```python
from build123d import *

# Parameters (mm, degrees)
SKETCH1_R           = 16
BOSS_EXTRUDE1_DEPTH = 7
CUT_EXTRUDE1_START  = -5
SKETCH3_R           = 16
SKETCH3_R_2         = 15
CUT_EXTRUDE1_DEPTH  = 5


with BuildPart() as part:
    # Sketch1 → Boss-Extrude1 (new body)
    with BuildSketch(Plane(origin=(0, 0, 0), x_dir=(0, 0, -1), z_dir=(1, 0, 0))):
        Circle(SKETCH1_R)
        with BuildLine():
            Line((-1.923932435, 0.546336878), (1.435107833, 1.393005925))
            ThreePointArc((1.435107833, 1.393005925), (0.488824602, -1.939342803), (-1.923932435, 0.546336878))
        make_face(mode=Mode.SUBTRACT)
    extrude(amount=BOSS_EXTRUDE1_DEPTH)

    # Sketch3 → Cut-Extrude1 (cut)
    with BuildSketch(Plane(origin=(6, 0, 0), x_dir=(0, 0, -1), z_dir=(1, 0, 0)).offset(CUT_EXTRUDE1_START)):
        Circle(SKETCH3_R)
        Circle(SKETCH3_R_2, mode=Mode.SUBTRACT)
    extrude(amount=CUT_EXTRUDE1_DEPTH, mode=Mode.SUBTRACT)


solid = part.part
```
The model under review builds one solid part; all positions refer to its coordinate system, in mm. A direction names the side the tool comes from. Round coordinates to 2 decimals unless told otherwise and drop trailing zeros. Order: outer loops, then holes, each group sorted by start corner. A loop starts at its lowest first (then second) coordinate and runs counter-clockwise, first axis right, second up. Notation, with made-up numbers: (-8.5, 89.5) -> (7.5, 89.5) arc R21 ccw to (7.5, 98.5) -> close; hole circle Ø10 at (28, -33). An arc over 180 degrees is marked (long way). Use a Markdown table: item, result.
Q1. Mouldability with a two-part tool opening along Y and no side actions: class faces 1 (the cylindrical face through (3.451, -1.924, -0.545)), 2 (the cylindrical face through (0.49, -15.62, 3.47)), 3 (the flat face through (7, 0, -3)) as +Y half, -Y half, draft (parallel to the pull), parting line (faces both ways), or undercut.
Values:
| item | result |
|---|---|
| face 1 | undercut |
| face 2 | parting line |
| face 3 | draft |
Q2. We need section C-C on z = 6.5. Write out the cut boundary in (x, y).
Values:
| item | result |
|---|---|
| outline | (0, -14.62) -> (1, -14.62) -> (1, -13.52) -> (6, -13.52) -> (6, -14.62) -> (7, -14.62) -> (7, 14.62) -> (6, 14.62) -> (6, 13.52) -> (1, 13.52) -> (1, 14.62) -> (0, 14.62) -> close |
Q3. We need section A-A on y = 0. Write out the cut boundary in (x, z), then the cut area to 3 significant figures.
Values:
| item | result |
|---|---|
| outline | (0, -16) -> (1, -16) -> (1, -15) -> (6, -15) -> (6, -16) -> (7, -16) -> (7, -2) -> (0, -2) -> close; (0, 2) -> (7, 2) -> (7, 16) -> (6, 16) -> (6, 15) -> (1, 15) -> (1, 16) -> (0, 16) -> close |
| area | 186 mm^2 |
Q4. We need section B-B on z = -1. Write out the cut boundary in (x, y), then the cut area to 3 significant figures.
Values:
| item | result |
|---|---|
| outline | (0, -15.97) -> (1, -15.97) -> (1, -14.97) -> (6, -14.97) -> (6, -15.97) -> (7, -15.97) -> (7, -1.73) -> (0, -1.73) -> close; (0, 1.28) -> (7, 1.28) -> (7, 15.97) -> (6, 15.97) -> (6, 14.97) -> (1, 14.97) -> (1, 15.97) -> (0, 15.97) -> close |
| area | 192 mm^2 |
Q5. For line 1 (X direction, y = -6, z = 14); line 2 (Y direction, x = 4.75, z = 0); line 3 (Z direction, x = 4, y = 9), list the stretches that pass through material, from the lowest coordinate up.
Values:
| item | result |
|---|---|
| line 1 | x = 0 to 1, 6 to 7 |
| line 2 | y = -15 to -2, 1.03 to 15 |
| line 3 | z = -12 to 12 |
Q6. Tool access review of faces 4 (the cylindrical face through (3.465, 0.66, 14.985)), 5 (the flat face through (0, 0, -3)), 6 (the flat face through (3.451, 0.964, 0.268)): name each direction out of +Z, -Z, +X, -X, +Y, -Y from which nothing blocks a thin tool from reaching the whole face with its end or side.
Values:
| item | result |
|---|---|
| face 4 | none |
| face 5 | +Z, -Z, -X, +Y, -Y |
| face 6 | +X, -X |
Q7. We need section D-D on y = -9. Write out the cut boundary in (x, z), then the cut area to 3 significant figures.
Values:
| item | result |
|---|---|
| outline | (0, -13.23) -> (1, -13.23) -> (1, -12) -> (6, -12) -> (6, -13.23) -> (7, -13.23) -> (7, 13.23) -> (6, 13.23) -> (6, 12) -> (1, 12) -> (1, 13.23) -> (0, 13.23) -> close |
| area | 173 mm^2 |
Q8. Clearance check with flat-ended pins moving along their axes: P1, Ø3, axis at x = 5.5, y = 12.5, coming from the +Z side; P2, Ø3, axis at x = 1.5, y = -2, coming from the -Z side; P3, Ø4.5, axis at y = 0, z = 0, coming from the -X side; P4, Ø2, axis at x = 2.5, z = -8, coming from the -Y side. State where each tip first meets the part, or that it passes through.
Values:
| item | result |
|---|---|
| P1 | stops at z = 11.54 |
| P2 | stops at z = -15.99 |
| P3 | stops at x = 0 |
| P4 | stops at y = -13.27 |
